```python
from build123d import *

# Parameters (mm, degrees)
BOSS_EXTRUDE1_DEPTH = 300


with BuildPart() as part:
    # Sketch1 → Boss-Extrude1 (new body)
    with BuildSketch(Plane.XY):
        with BuildLine():
            Line((-2.746356642, -3.807016814), (-5.847983186, -6.908643358))
            ThreePointArc((-5.847983186, -6.908643358), (-5.956791575, -7.07148662), (-5.995, -7.263573344))
            Line((-5.995, -7.263573344), (-5.995, -7.858053199))
            ThreePointArc((-5.995, -7.858053199), (-5.847983186, -8.212983186), (-5.493053199, -8.36))
            Line((-5.493053199, -8.36), (-3.131946801, -8.36))
            ThreePointArc((-3.131946801, -8.36), (-2.777016814, -8.507016814), (-2.63, -8.861946801))
            Line((-2.63, -8.861946801), (-2.63, -9.498053199))
            ThreePointArc((-2.63, -9.498053199), (-2.777016814, -9.852983186), (-3.131946801, -10))
            Line((-3.131946801, -10), (-8.5, -10))
            ThreePointArc((-8.5, -10), (-9.560660172, -9.560660172), (-10, -8.5))
            Line((-10, -8.5), (-10, -3.131946801))
            ThreePointArc((-10, -3.131946801), (-9.852983186, -2.777016814), (-9.498053199, -2.63))
            Line((-9.498053199, -2.63), (-8.861946801, -2.63))
            ThreePointArc((-8.861946801, -2.63), (-8.507016814, -2.777016814), (-8.36, -3.131946801))
            Line((-8.36, -3.131946801), (-8.36, -5.493053199))
            ThreePointArc((-8.36, -5.493053199), (-8.212983186, -5.847983186), (-7.858053199, -5.995))
            Line((-7.858053199, -5.995), (-7.263573344, -5.995))
            ThreePointArc((-7.263573344, -5.995), (-7.07148662, -5.956791575), (-6.908643358, -5.847983186))
            Line((-6.908643358, -5.847983186), (-3.807016814, -2.746356642))
            ThreePointArc((-3.807016814, -2.746356642), (-3.698208425, -2.58351338), (-3.66, -2.391426656))
            Line((-3.66, -2.391426656), (-3.66, 2.391426656))
            ThreePointArc((-3.66, 2.391426656), (-3.698208425, 2.58351338), (-3.807016814, 2.746356642))
            Line((-3.807016814, 2.746356642), (-6.908643358, 5.847983186))
            ThreePointArc((-6.908643358, 5.847983186), (-7.07148662, 5.956791575), (-7.263573344, 5.995))
            Line((-7.263573344, 5.995), (-7.858053199, 5.995))
            ThreePointArc((-7.858053199, 5.995), (-8.212983186, 5.847983186), (-8.36, 5.493053199))
            Line((-8.36, 5.493053199), (-8.36, 3.131946801))
            ThreePointArc((-8.36, 3.131946801), (-8.507016814, 2.777016814), (-8.861946801, 2.63))
            Line((-8.861946801, 2.63), (-9.498053199, 2.63))
            ThreePointArc((-9.498053199, 2.63), (-9.852983186, 2.777016814), (-10, 3.131946801))
            Line((-10, 3.131946801), (-10, 8.5))
            ThreePointArc((-10, 8.5), (-9.560660172, 9.560660172), (-8.5, 10))
            Line((-8.5, 10), (-3.131946801, 10))
            ThreePointArc((-3.131946801, 10), (-2.777016814, 9.852983186), (-2.63, 9.498053199))
            Line((-2.63, 9.498053199), (-2.63, 8.861946801))
            ThreePointArc((-2.63, 8.861946801), (-2.777016814, 8.507016814), (-3.131946801, 8.36))
            Line((-3.131946801, 8.36), (-5.493053199, 8.36))
            ThreePointArc((-5.493053199, 8.36), (-5.847983186, 8.212983186), (-5.995, 7.858053199))
            Line((-5.995, 7.858053199), (-5.995, 7.263573344))
            ThreePointArc((-5.995, 7.263573344), (-5.956791575, 7.07148662), (-5.847983186, 6.908643358))
            Line((-5.847983186, 6.908643358), (-2.746356642, 3.807016814))
            ThreePointArc((-2.746356642, 3.807016814), (-2.58351338, 3.698208425), (-2.391426656, 3.66))
            Line((-2.391426656, 3.66), (2.391426656, 3.66))
            ThreePointArc((2.391426656, 3.66), (2.58351338, 3.698208425), (2.746356642, 3.807016814))
            Line((2.746356642, 3.807016814), (5.847983186, 6.908643358))
            ThreePointArc((5.847983186, 6.908643358), (5.956791575, 7.07148662), (5.995, 7.263573344))
            Line((5.995, 7.263573344), (5.995, 7.858053199))
            ThreePointArc((5.995, 7.858053199), (5.847983186, 8.212983186), (5.493053199, 8.36))
            Line((5.493053199, 8.36), (3.131946801, 8.36))
            ThreePointArc((3.131946801, 8.36), (2.777016814, 8.507016814), (2.63, 8.861946801))
            Line((2.63, 8.861946801), (2.63, 9.498053199))
            ThreePointArc((2.63, 9.498053199), (2.777016814, 9.852983186), (3.131946801, 10))
            Line((3.131946801, 10), (8.5, 10))
            ThreePointArc((8.5, 10), (9.560660172, 9.560660172), (10, 8.5))
            Line((10, 8.5), (10, 3.131946801))
            ThreePointArc((10, 3.131946801), (9.852983186, 2.777016814), (9.498053199, 2.63))
            Line((9.498053199, 2.63), (8.861946801, 2.63))
            ThreePointArc((8.861946801, 2.63), (8.507016814, 2.777016814), (8.36, 3.131946801))
            Line((8.36, 3.131946801), (8.36, 5.493053199))
            ThreePointArc((8.36, 5.493053199), (8.212983186, 5.847983186), (7.858053199, 5.995))
            Line((7.858053199, 5.995), (7.263573344, 5.995))
            ThreePointArc((7.263573344, 5.995), (7.07148662, 5.956791575), (6.908643358, 5.847983186))
            Line((6.908643358, 5.847983186), (3.807016814, 2.746356642))
            ThreePointArc((3.807016814, 2.746356642), (3.698208425, 2.58351338), (3.66, 2.391426656))
            Line((3.66, 2.391426656), (3.66, -2.391426656))
            ThreePointArc((3.66, -2.391426656), (3.698208425, -2.58351338), (3.807016814, -2.746356642))
            Line((3.807016814, -2.746356642), (6.908643358, -5.847983186))
            ThreePointArc((6.908643358, -5.847983186), (7.07148662, -5.956791575), (7.263573344, -5.995))
            Line((7.263573344, -5.995), (7.858053199, -5.995))
            ThreePointArc((7.858053199, -5.995), (8.212983186, -5.847983186), (8.36, -5.493053199))
            Line((8.36, -5.493053199), (8.36, -3.131946801))
            ThreePointArc((8.36, -3.131946801), (8.507016814, -2.777016814), (8.861946801, -2.63))
            Line((8.861946801, -2.63), (9.498053199, -2.63))
            ThreePointArc((9.498053199, -2.63), (9.852983186, -2.777016814), (10, -3.131946801))
            Line((10, -3.131946801), (10, -8.5))
            ThreePointArc((10, -8.5), (9.560660172, -9.560660172), (8.5, -10))
            Line((8.5, -10), (3.131946801, -10))
            ThreePointArc((3.131946801, -10), (2.777016814, -9.852983186), (2.63, -9.498053199))
            Line((2.63, -9.498053199), (2.63, -8.861946801))
            ThreePointArc((2.63, -8.861946801), (2.777016814, -8.507016814), (3.131946801, -8.36))
            Line((3.131946801, -8.36), (5.493053199, -8.36))
            ThreePointArc((5.493053199, -8.36), (5.847983186, -8.212983186), (5.995, -7.858053199))
            Line((5.995, -7.858053199), (5.995, -7.263573344))
            ThreePointArc((5.995, -7.263573344), (5.956791575, -7.07148662), (5.847983186, -6.908643358))
            Line((5.847983186, -6.908643358), (2.746356642, -3.807016814))
            ThreePointArc((2.746356642, -3.807016814), (2.58351338, -3.698208425), (2.391426656, -3.66))
            Line((2.391426656, -3.66), (-2.391426656, -3.66))
            ThreePointArc((-2.391426656, -3.66), (-2.58351338, -3.698208425), (-2.746356642, -3.807016814))
        make_face()
        with BuildLine():
            ThreePointArc((-1.767678053, 0.935582333), (-2, 0), (-1.767678053, -0.935582333))
            ThreePointArc((-1.767678053, -0.935582333), (-1.834942097, -1.834942097), (-0.935582333, -1.767678053))
            ThreePointArc((-0.935582333, -1.767678053), (0, -2), (0.935582333, -1.767678053))
            ThreePointArc((0.935582333, -1.767678053), (1.834942097, -1.834942097), (1.767678053, -0.935582333))
            ThreePointArc((1.767678053, -0.935582333), (2, 0), (1.767678053, 0.935582333))
            ThreePointArc((1.767678053, 0.935582333), (1.834942097, 1.834942097), (0.935582333, 1.767678053))
            ThreePointArc((0.935582333, 1.767678053), (0, 2), (-0.935582333, 1.767678053))
            ThreePointArc((-0.935582333, 1.767678053), (-1.834942097, 1.834942097), (-1.767678053, 0.935582333))
        make_face(mode=Mode.SUBTRACT)
    extrude(amount=BOSS_EXTRUDE1_DEPTH)


solid = part.part
```
Verification items for the finished model (mm, model axes). A direction names the side the tool comes from. Give positions to 0.01 mm unless a question says otherwise; leave off trailing zeros. Put each result on its own line as item: value.
Q1. Mould release check, pull along Y, two halves, no side actions. Record for faces 4 (the face through (-6, -10, 148)), 5 (the face through (0.1, 2.4, 0)), 6 (the face through (0, 3.66, 148)), 7 (the face through (-3.66, 0, 148)): released by +Y, released by -Y, zero draft, split by the parting line, or undercut.
Result:
face 4: released by -Y
face 5: zero draft
face 6: released by +Y
face 7: undercut
Q2. Scan lines: probe 1 along X at (y, z) = (4.75, 81.5); probe 2 along X at (y, z) = (0.25, 170); probe 3 along X at (y, z) = (3.75, 202). Record each from-to range of solid material in increasing order. Write a range as from..to.
Result:
probe 1: -10..-8.36, -5.81..-3.69, 3.69..5.81, 8.36..10
probe 2: -3.66..-1.98, 1.98..3.66
probe 3: -10..-8.36, -4.81..-2.68, 2.68..4.81, 8.36..10
Q3. Depth check by flat-ended pin: P1, Ø4, axis at y = -0.5, z = 138, coming from the +X side; P2, Ø4, axis at y = 0.5, z = 170, coming from the -X side; P3, Ø0.5, axis at y = 9, z = 82, coming from the +X side; P4, Ø1, axis at x = -1.41, y = 1.41, coming from the +Z side. Enter the tip coordinate at first touch or a pass-through.
Result:
P1: x = 3.67
P2: x = -3.67
P3: x = 9.98
P4: through
Q4. Set-up check for faces 1 (the face through (0, -3.66, 148)), 2 (the face through (3.66, 0, 148)), 3 (the face through (-10, 6, 148)): record each of +Z, -Z, +X, -X, +Y, -Y from which the full face is reachable in a straight line by a thin tool's end or side.
Result:
face 1: +Z, -Z, -Y
face 2: +Z, -Z, +X
face 3: +Z, -Z, -X, +Y, -Y
